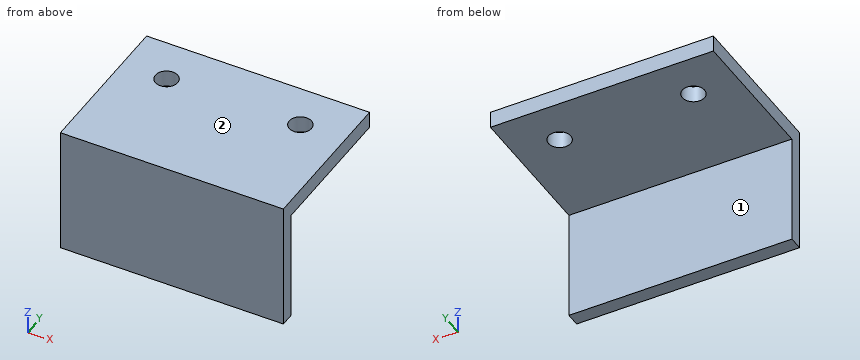
```python
from build123d import *

# Parameters (mm, degrees)
SKETCH002_W     = 40
SKETCH002_H     = 28
PAD_DEPTH       = 3
SKETCH_R        = 2
POCKET_DEPTH    = 5
SKETCH001_R     = 2
POCKET001_DEPTH = 5
SKETCH003_W     = 40
SKETCH003_H     = 2.5
PAD001_DEPTH    = 20


with BuildPart() as part:
    # Sketch002 → Pad (new body)
    with BuildSketch(Plane.XY):
        with Locations((12, -6)):
            Rectangle(SKETCH002_W, SKETCH002_H)
    extrude(amount=PAD_DEPTH)

    # Sketch → Pocket (cut)
    with BuildSketch(Plane.XY):
        Circle(SKETCH_R)
    extrude(amount=POCKET_DEPTH, mode=Mode.SUBTRACT)

    # Sketch001 → Pocket001 (cut)
    with BuildSketch(Plane.XY):
        with Locations((24, 0)):
            Circle(SKETCH001_R)
    extrude(amount=POCKET001_DEPTH, mode=Mode.SUBTRACT)

    # Sketch003 → Pad001 (join)
    with BuildSketch(Plane.XY):
        with Locations((12, -18.75)):
            Rectangle(SKETCH003_W, SKETCH003_H)
    extrude(amount=-PAD001_DEPTH)


solid = part.part
```
Build history of the part. All positions in model axes, mm. Face numbers are marked on the shaded views. A direction names the side the tool comes from. Give positions to 0.01 mm unless a question says otherwise; leave off trailing zeros. Loops run counter-clockwise (first coordinate to the right, second up) from the corner with the lowest first, then second, coordinate; pieces in that order, holes last.
1) 3-axis set-ups, long thin cutter, end or side, ignore diameter. For the marked faces 1 and 2: which of +Z, -Z, +X, -X, +Y, -Y reach the whole face in a straight line?
Values follow:
face 1: -Z, +X, -X, +Y
face 2: +Z, +X, -X, +Y, -Y
2) Band-saw the part on B-B on x = 24. List the corners of the cut face in (y, z).
Values follow:
outline: (-20, -20) - (-17.5, -20) - (-17.5, 0) - (-2, 0) - (-2, 3) - (-20, 3) - close; (2, 0) - (8, 0) - (8, 3) - (2, 3) - close
3) Band-saw the part on C-C on x = 12. List the corners of the cut face in (y, z), then the cut area to 3 significant figures.
Values follow:
outline: (-20, -20) - (-17.5, -20) - (-17.5, 0) - (8, 0) - (8, 3) - (-20, 3) - close
area: 134 mm2
4) Band-saw the part on A-A on y = 0. List the corners of the cut face in (x, z), then the cut area to 3 significant figures.
Values follow:
outline: (-8, 0) - (-2, 0) - (-2, 3) - (-8, 3) - close; (2, 0) - (22, 0) - (22, 3) - (2, 3) - close; (26, 0) - (32, 0) - (32, 3) - (26, 3) - close
area: 96.0 mm2
5) Probe line 1 along X through (y, z) = (0, 0.85); line 2 along Y through (x, z) = (24, 1.9); line 3 along Y through (x, z) = (6, -17.75). List the from-to ranges inside material, lowest first.
Values follow:
line 1: x = -8 to -2, 2 to 22, 26 to 32
line 2: y = -20 to -2, 2 to 8
line 3: y = -20 to -17.5
6) Drop flat-ended pins along their axis: P1, Ø7.5, axis at x = 15.5, y = -4.5, coming from the -Z side; P2, Ø2, axis at y = -7, z = -0.5, coming from the +X side; P3, Ø3.5, axis at x = 0, y = 0, coming from the -Z side. Give the stop position or say it passes through.
Values follow:
P1: stops at z = 0
P2: stops at x = 32
P3: passes through
7) Band-saw the part on D-D on z = -17. List the corners of the cut face in (x, y).
Values follow:
outline: (-8, -20) - (32, -20) - (32, -17.5) - (-8, -17.5) - close
